The listing builds one solid part. Answer for the finished solid, in the listing's coordinates (mm). A direction names the side the tool comes from. Give positions to 0.01 mm unless a question says otherwise; leave off trailing zeros. Write each loop counter-clockwise with the first axis right and the second up, starting at its lowest first coordinate (ties: lowest second). Pieces come first, ordered by that corner, then holes. Notation, with made-up numbers: (46, 17) - (54, 17) arc R27 cw to (54, 40) - close; hole circle Ø6 at (-5, -13). An arc over 180 degrees is marked (long way). Write each question's results on one line, items separated by ' | '. Start each with the question number.
Q1. Section D-D (z = -18) is taken. Determine the outline of the cut face in (x, y), plus the area to 3 significant figures.
Q2. Find the intervals of material crossed by probe 1 along Z at (x, y) = (5.9, -2.2); probe 2 along Z at (x, y) = (8, -0.75); probe 3 along Z at (x, y) = (21.25, -6.5), in increasing order.
Q3. For a pull along Z with two mould halves and no side action, classify faces 5 (the face through (17, -6, -57.2)), 6 (the face through (0.9, -2.97, -30.94)), 7 (the face through (24.8, -5, -33)) as pulls with the +Z half, pulls with the -Z half, needs draft (parallel to the pull), parting line crosses it, or undercut.
Q4. Section A-A (y = -5.75) is taken. Determine the outline of the cut face in (x, z), plus the area to 3 significant figures.
Q5. For faces 1 (the face through (14.8, -5, -54)), 2 (the face through (18.4, -3, -51)), 3 (the face through (19, -7, -49.9)), 4 (the face through (5.27, -2.46, -28.73)), determine the directions among +Z, -Z, +X, -X, +Y, -Y from which every point of the face is accessible in a straight line to the end or side of a thin tool.
Q6. Flat-ended cylindrical pins translate along their axes: pin 1 Ø1.8 at (x, y) = (16.5, -5) entering from -Z; pin 2 Ø3 at (x, y) = (10, -3.5) entering from -Z; pin 3 Ø12 at (x, z) = (5, -17) entering from -Y. Find the tip coordinate at first contact, or state that the pin passes through.
Q7. Section C-C (x = 5.9) is taken. Determine the outline of the cut face in (y, z).
Q8. Section B-B (z = -25.9) is taken. Determine the outline of the cut face in (x, y).
```python
from build123d import *

# Parameters (mm, degrees)
F0_R        = 2.9
F0_W        = 10
F0_H        = 34.1
F1_DEPTH    = 5
F2_W        = 10
F2_H        = 3
F3_DEPTH    = 6
F4_W        = 3.6
F4_H        = 3.6
F5_DEPTH    = 6
F6_W        = 3.6
F6_H        = 2.1
F6_H_2      = 1.6
F7_DEPTH    = 5.001
F8_T1_DEPTH = 20
F8_T3_DEPTH = 26
F9_R        = 1


# Not quite as in the source:
# - a fillet or chamfer that OpenCascade refuses, or shapes differently, is made with other operations: its cross-section is extruded or revolved along the edge and cut away or added


with BuildPart() as f1:
    # F0 (on Front) → F1 (new body)
    with BuildSketch(Plane.XZ):
        Polygon((24.8, 0), (0, 0), (0, -31.8), (14.8, -31.8), (24.8, -31.8), align=None)
        with Locations((5.9, -25.9)):
            Circle(F0_R, mode=Mode.SUBTRACT)
        with Locations((5.9, -5.9)):
            Circle(F0_R, mode=Mode.SUBTRACT)
        with Locations((19.8, -48.85)):
            Rectangle(F0_W, F0_H)
    extrude(amount=F1_DEPTH)

    # F2 (on face) → F3 (join)
    with BuildSketch(Plane.XZ.offset(5)):
        Polygon((14.8, -49.9), (24.8, -49.9), (24.8, 0), (14.8, 0), (14.8, -31.8), align=None)
        with Locations((19.8, -64.4)):
            Rectangle(F2_W, F2_H)
    extrude(amount=F3_DEPTH)

    # F4 (on face) → F5 (join, through all)
    with BuildSketch(Plane.XZ.offset(5)):
        with Locations((16.6, -53.8)):
            Rectangle(F4_W, F4_H)
        with Locations((16.6, -59)):
            Rectangle(F4_W, F4_H)
    extrude(amount=F5_DEPTH)

    # F6 (on face) → F7 (cut, through all)
    with BuildSketch(Plane.XZ.offset(5)):
        with Locations((16.6, -50.95)):
            Rectangle(F6_W, F6_H)
        with Locations((16.6, -56.4)):
            Rectangle(F6_W, F6_H_2)
        with Locations((16.6, -61.85)):
            Rectangle(F6_W, F6_H)
    extrude(amount=-F7_DEPTH, mode=Mode.SUBTRACT)

    # F8: fillet of radius 3 on 5 edges, made by hand

    # F8_s2 → F8_t1 (cut)
    with BuildSketch(Plane.XZ.offset(-7.5)):
        with BuildLine():
            ThreePointArc((3, -31.8), (0.8786796564, -30.9213203436), (0, -28.8))
            Line((0, -28.8), (0, -31.8))
            Line((0, -31.8), (3, -31.8))
        make_face()
        with BuildLine():
            ThreePointArc((3, 0), (0.8786796564, -0.8786796564), (0, -3))
            Line((0, -3), (0, 0))
            Line((0, 0), (3, 0))
        make_face()
    extrude(amount=F8_T1_DEPTH, mode=Mode.SUBTRACT)

    # F8_s4 → F8_t3 (cut)
    with BuildSketch(Plane.XZ.offset(-7.5)):
        with BuildLine():
            ThreePointArc((21.8, 0), (23.9213203436, -0.8786796564), (24.8, -3))
            Line((24.8, -3), (24.8, 0))
            Line((24.8, 0), (21.8, 0))
        make_face()
        with BuildLine():
            ThreePointArc((21.8, -65.9), (23.9213203436, -65.0213203436), (24.8, -62.9))
            Line((24.8, -62.9), (24.8, -65.9))
            Line((24.8, -65.9), (21.8, -65.9))
        make_face()
        with BuildLine():
            ThreePointArc((14.8, -62.9), (15.6786796564, -65.0213203436), (17.8, -65.9))
            Line((17.8, -65.9), (14.8, -65.9))
            Line((14.8, -65.9), (14.8, -62.9))
        make_face()
    extrude(amount=F8_T3_DEPTH, mode=Mode.SUBTRACT)

    # F9
    f9_edges = [f1.edges().sort_by_distance(p)[0] for p in [
        (14.8, 0, -53.8),
        (14.8, 0, -59),
        (14.8, 0, -40.85),
        (24.8, -11, -26.45),
        (15.67868, 0, -65.02132),
        (14.8, -11, -24.95),
        (23.92132, -11, -65.02132),
        (12.4, 0, 0),
        (18.3, -11, 0),
        (23.92132, 0, -0.87868),
        (23.92132, -11, -0.87868),
        (8.9, 0, -31.8),
        (0.87868, 0, -30.92132),
        (0, 0, -15.9),
        (0.87868, 0, -0.87868),
        (24.8, 0, -32.95),
        (23.92132, 0, -65.02132),
        (19.8, 0, -65.9),
        (15.67868, -11, -65.02132),
        (14.8, -11, -59),
        (14.8, -11, -53.8),
        (19.8, -11, -65.9),
    ]]
    fillet(f9_edges, radius=F9_R)


solid = f1.part
```
Answers below:
1) outline: (0, -5) - (14.8, -5) - (14.8, -10) arc R1 ccw to (15.8, -11) - (23.8, -11) arc R1 ccw to (24.8, -10) - (24.8, -1) arc R1 ccw to (23.8, 0) - (1, 0) arc R1 ccw to (0, -1) - close | area: 183 mm2
2) probe 1: z = -31.8 to -28.8, -23 to -8.8, -3 to 0 | probe 2: z = -31.77 to -27.9, -23.9 to -7.9, -3.9 to -0.03 | probe 3: z = -65.9 to -62.9, -49.9 to 0
3) face 5: undercut | face 6: pulls with the -Z half | face 7: needs draft
4) outline: (14.8, -62.9) arc R3 ccw to (17.8, -65.9) - (21.8, -65.9) arc R3 ccw to (24.8, -62.9) - close; (14.8, -60.8) - (18.4, -60.8) - (18.4, -57.2) - (14.8, -57.2) - close; (14.8, -55.6) - (18.4, -55.6) - (18.4, -52) - (14.8, -52) - close; (14.8, -49.9) - (24.8, -49.9) - (24.8, -3) arc R3 ccw to (21.8, 0) - (14.8, 0) - close | area: 549 mm2
5) face 1: -Z, -X, +Y, -Y | face 2: -X, +Y, -Y | face 3: -X, -Y | face 4: +Y, -Y
6) pin 1: stops at z = -65.87 | pin 2: stops at z = -31.8 | pin 3: stops at y = -5
7) outline: (-5, -31.8) - (-1, -31.8) arc R1 ccw to (0, -30.8) - (0, -28.8) - (-5, -28.8) - close; (-5, -23) - (0, -23) - (0, -8.8) - (-5, -8.8) - close; (-5, -3) - (0, -3) - (0, -1) arc R1 ccw to (-1, 0) - (-5, 0) - close
8) outline: (0, -5) - (3, -5) - (3, 0) - (1, 0) arc R1 ccw to (0, -1) - close; (8.8, -5) - (14.8, -5) - (14.8, -10) arc R1 ccw to (15.8, -11) - (23.8, -11) arc R1 ccw to (24.8, -10) - (24.8, -1) arc R1 ccw to (23.8, 0) - (8.8, 0) - close
